Design review of the part built by this model. Coordinates are the model's own, in mm. Face numbers are marked on the shaded views. A direction names the side the tool comes from. Coordinates: 2 decimals unless noted, no trailing zeros. Order: outer loops, then holes, each group sorted by start corner. A loop starts at its lowest first (then second) coordinate and runs counter-clockwise, first axis right, second up. Notation, with made-up numbers: M 89,-32.5 L 121,-32.5 A19 cw 121,-13.5 Z; hole C 33.25,-26.5 d6. An arc over 180 degrees is marked long. Answer in a Markdown table with one row per item.
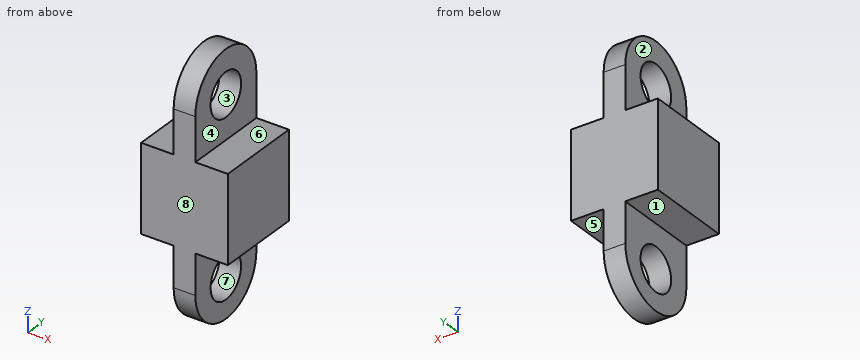
from build123d import *

# Parameters (mm, degrees)
F0_W     = 40
F0_H     = 40
F1_DEPTH = 40
F3_DEPTH = 5
F4_R     = 10
F5_DEPTH = 25


with BuildPart() as f1:
    # F0 (on Top) → F1 (new body)
    with BuildSketch(Plane.XY):
        Rectangle(F0_W, F0_H)
    extrude(amount=F1_DEPTH)

    # F2 (on Right) → F3 (join, symmetric)
    with BuildSketch(Plane.YZ):
        with BuildLine():
            Line((-20, 60), (-20, 40))
            Line((-20, 40), (20, 40))
            Line((20, 40), (20, 60))
            ThreePointArc((20, 60), (0, 80), (-20, 60))
        make_face()
        with BuildLine():
            Line((20, -18.422272), (20, 0))
            Line((20, 0), (-20, 0))
            Line((-20, 0), (-20, -18.422272))
            ThreePointArc((-20, -18.422272), (0, -38.422272), (20, -18.422272))
        make_face()
    extrude(amount=F3_DEPTH, both=True)

    # F4 (on face) → F5 (cut)
    with BuildSketch(Plane.YZ.offset(5)):
        with Locations((0, 60)):
            Circle(F4_R)
        with Locations((0, -20)):
            Circle(F4_R)
    extrude(amount=-F5_DEPTH, mode=Mode.SUBTRACT)


solid = f1.part
(1) Add section D-D, the plane y = -5.5. Give the boundary of the cut face in (x, z).
Return value:
| item | result |
|---|---|
| outline | M -20,0 L -5,0 L -5,-11.65 L 5,-11.65 L 5,0 L 20,0 L 20,40 L 5,40 L 5,51.65 L -5,51.65 L -5,40 L -20,40 Z; M -5,-37.65 L 5,-37.65 L 5,-28.35 L -5,-28.35 Z; M -5,68.35 L 5,68.35 L 5,79.23 L -5,79.23 Z |
(2) Add section A-A, the plane y = 0. Give the boundary of the cut face in (x, z).
Return value:
| item | result |
|---|---|
| outline | M -20,0 L -5,0 L -5,-10 L 5,-10 L 5,0 L 20,0 L 20,40 L 5,40 L 5,50 L -5,50 L -5,40 L -20,40 Z; M -5,-38.42 L 5,-38.42 L 5,-30 L -5,-30 Z; M -5,70 L 5,70 L 5,80 L -5,80 Z |
(3) Add section B-B, the plane z = -23.5. Give the boundary of the cut face in (x, y).
Return value:
| item | result |
|---|---|
| outline | M -5,-19.34 L 5,-19.34 L 5,-9.37 L -5,-9.37 Z; M -5,9.37 L 5,9.37 L 5,19.34 L -5,19.34 Z |
(4) For line 1 along Z through (x, y) = (1.25, 0); line 2 along Z through (x, y) = (-11.5, -4.5); line 3 along X through (y, z) = (-12.5, -8.5), list the stretches that pass through material, from the lowest coordinate up. Write a range as from..to.
Return value:
| item | result |
|---|---|
| line 1 | z = -38.42..-30, -10..50, 70..80 |
| line 2 | z = 0..40 |
| line 3 | x = -5..5 |
(5) Add section C-C, the plane x = 12.5. Give the boundary of the cut face in (y, z), and give its area (3 significant figures).
Return value:
| item | result |
|---|---|
| outline | M -20,0 L 20,0 L 20,40 L -20,40 Z |
| area | 1,600 mm2 |
(6) Insertion check: pin 1 Ø12 at (x, y) = (13, 3.5) entering from -Z; pin 2 Ø12 at (y, z) = (5.5, 51) entering from -X; pin 3 Ø1.5 at (y, z) = (-11.5, 55.5) entering from +X; pin 4 Ø12 at (y, z) = (0, -20) entering from +X. Each pin has a flat end and moves straight along its axis. Give the tip position at first contact, or say it passes through.
Return value:
| item | result |
|---|---|
| pin 1 | stops at z = 0 |
| pin 2 | stops at x = -5 |
| pin 3 | stops at x = 5 |
| pin 4 | passes through |
(7) For the marked faces 1, 2, 3, 4 and 5, list the 3-axis set-ups (+Z, -Z, +X, -X, +Y, -Y) from which the entire face can be reached by the end or side of a thin tool; tool diameter is ignored.
Return value:
| item | result |
|---|---|
| face 1 | -Z, -X, +Y, -Y |
| face 2 | +Z, -X, +Y, -Y |
| face 3 | +X, -X |
| face 4 | +Z, +X, +Y, -Y |
| face 5 | -Z, +X, +Y, -Y |
(8) Draft analysis for pull direction Z (two halves, no side actions). For the marked faces 6, 7 and 8, state which applies: pulls with the +Z half, pulls with the -Z half, needs draft (parallel to the pull), parting line crosses it, or undercut.
Return value:
| item | result |
|---|---|
| face 6 | pulls with the +Z half |
| face 7 | undercut |
| face 8 | needs draft |
